from build123d import *

# Parameters (mm, degrees)
SKETCH1_W                = 18
SKETCH1_H                = 18
BOSS_EXTRUDE1_DEPTH      = 2
SKETCH2_W                = 2.5
SKETCH2_H                = 10
BOSS_EXTRUDE2_DEPTH      = 3
BOSS_EXTRUDE3_DEPTH      = 6
BOSS_EXTRUDE3_DEPTH_BACK = 6
SKETCH3_W                = 0.5
SKETCH3_H                = 8


with BuildPart() as part:
    # Sketch1 → Boss-Extrude1 (new body)
    with BuildSketch(Plane(origin=(0, 0, 0), x_dir=(1, 0, 0), z_dir=(0, 1, 0))):
        Rectangle(SKETCH1_W, SKETCH1_H)
    extrude(amount=BOSS_EXTRUDE1_DEPTH)

    # Sketch2 → Boss-Extrude2 (add)
    with BuildSketch(Plane(origin=(0, 2, 0), x_dir=(1, 0, 0), z_dir=(0, 1, 0))):
        with Locations((-7.75, 0)):
            Rectangle(SKETCH2_W, SKETCH2_H)
        with Locations((7.75, 0)):
            Rectangle(SKETCH2_W, SKETCH2_H)
    extrude(amount=BOSS_EXTRUDE2_DEPTH)

    # Sketch3 → Boss-Extrude3 (add, two sides: drawn at the far end of the back side and taken through both)
    with BuildSketch(Plane(origin=(0, 5, 0), x_dir=(1, 0, 0), z_dir=(0, 1, 0)).offset(-BOSS_EXTRUDE3_DEPTH_BACK)):
        with Locations((-7.887555613, 0)):
            Rectangle(SKETCH3_W, SKETCH3_H)
        with Locations((7.887555613, 0)):
            Rectangle(SKETCH3_W, SKETCH3_H)
    extrude(amount=BOSS_EXTRUDE3_DEPTH + BOSS_EXTRUDE3_DEPTH_BACK)


solid = part.part
Input: part model. Units: mm. Frame: model coordinates. A direction names the side the tool comes from. Give positions to 0.01 mm unless a question says otherwise; leave off trailing zeros. Loops run counter-clockwise (first coordinate to the right, second up) from the corner with the lowest first, then second, coordinate; pieces in that order, holes last. Notation, with made-up numbers: M 84,3.5 L 126,3.5 A22 cw 126,40.5 Z; hole C 30,11.25 d1. An arc over 180 degrees is marked long. Use CSV: the item, a comma, the result in double quotes.
(1) Section B-B, the plane x = -7.25. Return loops of the section in (y, z).
Outcome:
outline,"M 0,-9 L 2,-9 L 2,-5 L 5,-5 L 5,5 L 2,5 L 2,9 L 0,9 Z"
(2) Section A-A, the plane y = 3. Return loops of the section in (x, z).
Outcome:
outline,"M -9,-5 L -6.5,-5 L -6.5,5 L -9,5 Z; M 6.5,-5 L 9,-5 L 9,5 L 6.5,5 Z"
(3) Section C-C, the plane z = -2.5. Return loops of the section in (x, y), plus the area to 3 significant figures.
Outcome:
outline,"M -9,0 L -8.14,0 L -8.14,-1 L -7.64,-1 L -7.64,0 L 7.64,0 L 7.64,-1 L 8.14,-1 L 8.14,0 L 9,0 L 9,5 L 8.14,5 L 8.14,11 L 7.64,11 L 7.64,5 L 6.5,5 L 6.5,2 L -6.5,2 L -6.5,5 L -7.64,5 L -7.64,11 L -8.14,11 L -8.14,5 L -9,5 Z"
area,"58.0 mm²"
(4) Section D-D, the plane y = 5.75. Return loops of the section in (x, z).
Outcome:
outline,"M -8.14,-4 L -7.64,-4 L -7.64,4 L -8.14,4 Z; M 7.64,-4 L 8.14,-4 L 8.14,4 L 7.64,4 Z"
(5) Material intervals for L1, parallel to X at y = 2.25, z = -2.25; L2, parallel to X at y = 6.25, z = 1.5; L3, parallel to Y at x = -2.75, z = -4.5, sorted ascending. Write a range as [from, to].
Outcome:
L1,"x = [-9, -6.5], [6.5, 9]"
L2,"x = [-8.14, -7.64], [7.64, 8.14]"
L3,"y = [0, 2]"
(6) Pin query (flat end, axial travel): P1, Ø2, axis at x = -7.5, y = 3.5, coming from the +Z side; P2, Ø0.6, axis at x = -8, y = -0.5, coming from the +Z side; P3, Ø1.8, axis at y = 9, z = 1, coming from the +X side. Return the tip coordinate at first contact, or that it passes through.
Outcome:
P1,"stops at z = 5"
P2,"stops at z = 4"
P3,"stops at x = 8.14"
(7) Pull-direction query (X, two-part tool) for faces 1 (the face through (0, 0, 0)), 2 (the face through (-8, 3, -5)), 3 (the face through (-8.138, -0.5, 0.1)); classes: pulls with the +X half, pulls with the -X half, needs draft (parallel to the pull), parting line crosses it, or undercut.
Outcome:
face 1,"undercut"
face 2,"needs draft"
face 3,"pulls with the -X half"
(8) Set-up query: faces 4 (the face through (6.5, 3, 0)), 5 (the face through (7.638, -0.5, 0.1)), 6 (the face through (8, 3, -5)). Return all of +Z, -Z, +X, -X, +Y, -Y with unobstructed straight access to the full face (end or side cutting, diameter ignored); none if empty.
Outcome:
face 4,"+Z, -Z, +Y"
face 5,"+Z, -Z, -Y"
face 6,"-Z, +X, -X, +Y"
